from build123d import *

# Parameters (mm, degrees)
BOSS_EXTRUDE1_DEPTH      = 2
BOSS_EXTRUDE1_DEPTH_BACK = 3
SKETCH1_R                = 3.25
SKETCH2_R                = 14
BOSS_EXTRUDE2_DEPTH      = 3
SKETCH3_R                = 2.6
BOSS_EXTRUDE3_DEPTH      = 4.5
FILLET1_R                = 0.5


with BuildPart() as part:
    # Sketch1 → Boss-Extrude1 (new, two sides: drawn at the far end of the back side and taken through both)
    with BuildSketch(Plane.XY.offset(-BOSS_EXTRUDE1_DEPTH_BACK)):
        with Locations((17.35, 0)):
            Circle(SKETCH1_R)
    extrude(amount=BOSS_EXTRUDE1_DEPTH + BOSS_EXTRUDE1_DEPTH_BACK)

    # Sketch2 → Boss-Extrude2 (add)
    with BuildSketch(Plane.XY.offset(2)):
        with Locations((17.35, 0)):
            Circle(SKETCH2_R)
    extrude(amount=BOSS_EXTRUDE2_DEPTH)

    # Sketch3 → Boss-Extrude3 (add)
    with BuildSketch(Plane(origin=(0, 0, -3), x_dir=(-1, 0, 0), z_dir=(0, 0, -1))):
        with Locations((-17.35, 0)):
            Circle(SKETCH3_R)
    extrude(amount=BOSS_EXTRUDE3_DEPTH)

    # Fillet1
    fillet1_edges = [part.edges().sort_by_distance(p)[0] for p in [
        (19.95, 0, -7.5),
        (14.1, 0, 2),
        (3.35, 0, 2),
        (3.35, 0, 5),
    ]]
    fillet(fillet1_edges, radius=FILLET1_R)


solid = part.part
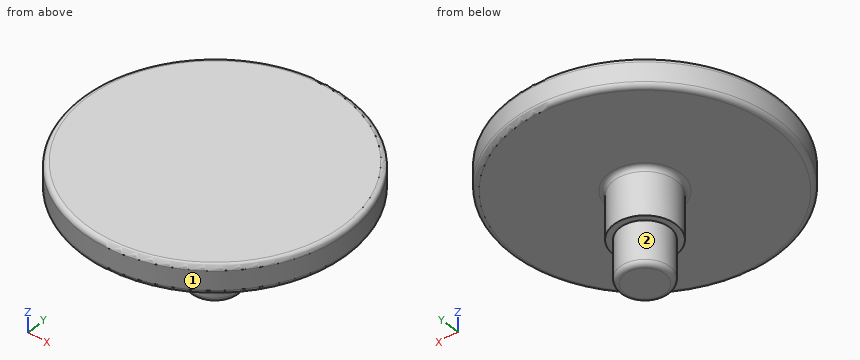
Read the model definition and answer for the solid it produces. Units are mm, in the model's axes. Face numbers are marked on the shaded views. A direction names the side the tool comes from. Coordinates: 2 decimals unless noted, no trailing zeros. Order: outer loops, then holes, each group sorted by start corner. A loop starts at its lowest first (then second) coordinate and runs counter-clockwise, first axis right, second up. Notation, with made-up numbers: M 27,26 L 49,26 A30 ccw 49,54 Z; hole C -36,89.25 d6. An arc over 180 degrees is marked long. Put each result on its own line as item: value. Start each with the question number.
Item 1: For the marked faces 1 and 2, determine the directions among +Z, -Z, +X, -X, +Y, -Y from which every point of the face is accessible in a straight line to the end or side of a thin tool.
Item 2: Consider probe 1 along Y at (x, z) = (17.5, 1); probe 2 along Z at (x, y) = (18.25, -8.75); probe 3 along Y at (x, z) = (20, -2.75). Determine where each line is inside the solid, lowest interval first. Write a range as [from, to].
Item 3: Section A-A, the plane y = 0 is taken. Determine the outline of the cut face in (x, z), plus the area to 3 significant figures.
Item 4: Section C-C, the plane z = -4.5 is taken. Determine the outline of the cut face in (x, y), plus the area to 3 significant figures.
Item 5: Section D-D, the plane z = 3.75 is taken. Determine the outline of the cut face in (x, y), plus the area to 3 significant figures.
Item 6: Given pin 1 Ø3 at (x, y) = (27.5, 5) entering from -Z; pin 2 Ø3 at (x, z) = (9.5, -1) entering from -Y, each flat-ended and moving along its own axis, determine where each tip first touches the part or whether it passes through.
Item 7: Section B-B, the plane x = 17.35 is taken. Determine the outline of the cut face in (y, z), plus the area to 3 significant figures.
Computed:
1. face 1: +Z, -Z
1. face 2: -Z
2. probe 1: y = [-3.25, 3.25]
2. probe 2: z = [2, 5]
2. probe 3: y = [-1.88, 1.88]
3. outline: M 3.35,2.5 A0.5 ccw 3.85,2 L 13.6,2 A0.5 cw 14.1,1.5 L 14.1,-3 L 14.75,-3 L 14.75,-7 A0.5 ccw 15.25,-7.5 L 19.45,-7.5 A0.5 ccw 19.95,-7 L 19.95,-3 L 20.6,-3 L 20.6,1.5 A0.5 cw 21.1,2 L 30.85,2 A0.5 ccw 31.35,2.5 L 31.35,4.5 A0.5 ccw 30.85,5 L 3.85,5 A0.5 ccw 3.35,4.5 Z
3. area: 140 mm2
4. outline: C 17.35,0 d5.2
4. area: 21.2 mm2
5. outline: C 17.35,0 d28
5. area: 616 mm2
6. pin 1: stops at z = 2
6. pin 2: passes through
7. outline: M -14,2.5 A0.5 ccw -13.5,2 L -3.75,2 A0.5 cw -3.25,1.5 L -3.25,-3 L -2.6,-3 L -2.6,-7 A0.5 ccw -2.1,-7.5 L 2.1,-7.5 A0.5 ccw 2.6,-7 L 2.6,-3 L 3.25,-3 L 3.25,1.5 A0.5 cw 3.75,2 L 13.5,2 A0.5 ccw 14,2.5 L 14,4.5 A0.5 ccw 13.5,5 L -13.5,5 A0.5 ccw -14,4.5 Z
7. area: 140 mm2
